Verification items for the finished model (mm, model axes). A direction names the side the tool comes from. Round coordinates to 2 decimals unless told otherwise and drop trailing zeros. Write each loop counter-clockwise with the first axis right and the second up, starting at its lowest first coordinate (ties: lowest second). Pieces come first, ordered by that corner, then holes. Notation, with made-up numbers: M 18,79 L 71,79 A12 ccw 71,83 Z; hole C 37,-33 d4. An arc over 180 degrees is marked long. One line per question, with ' | ' between items.
from build123d import *

# Parameters (mm, degrees)
SKETCH1_R           = 10
BOSS_EXTRUDE1_DEPTH = 4
SKETCH2_W           = 80
SKETCH2_H           = 30
BOSS_EXTRUDE2_DEPTH = 4
SKETCH5_W           = 15
SKETCH5_H           = 25.341978046
SKETCH5_R           = 3.5
BOSS_EXTRUDE3_DEPTH = 4
CUT_EXTRUDE1_DEPTH  = 5
SKETCH7_R           = 3.25
CUT_EXTRUDE2_DEPTH  = 5
LPATTERN1_COUNT     = 4
LPATTERN1_PITCH     = 12
SKETCH8_W           = 65
SKETCH8_H           = 10
BOSS_EXTRUDE4_DEPTH = 4
SKETCH9_R           = 1.175
CUT_EXTRUDE3_DEPTH  = 4
SKETCH10_W          = 10
SKETCH10_H          = 25
BOSS_EXTRUDE5_DEPTH = 4
SKETCH11_R          = 1.175
CUT_EXTRUDE4_DEPTH  = 4
SKETCH12_R          = 1
CUT_EXTRUDE5_DEPTH  = 5
CIRPATTERN1_COUNT   = 4
SKETCH13_R          = 3.5
CUT_EXTRUDE6_DEPTH  = 5
FILLET1_R           = 2


with BuildPart() as part:
    # Sketch1 → Boss-Extrude1 (new body)
    with BuildSketch(Plane(origin=(0, 0, 0), x_dir=(1, 0, 0), z_dir=(0, 1, 0))):
        Circle(SKETCH1_R)
    extrude(amount=BOSS_EXTRUDE1_DEPTH)

    # Sketch2 → Boss-Extrude2 (add)
    with BuildSketch(Plane(origin=(0, 0, 0), x_dir=(1, 0, 0), z_dir=(0, 1, 0))):
        with Locations((-40, 0)):
            Rectangle(SKETCH2_W, SKETCH2_H)
        Polygon((7.453553273, 6.666674104), (7.453553273, -6.666674104), (0, -15), (0, 15), align=None)
    extrude(amount=BOSS_EXTRUDE2_DEPTH)

    # Sketch5 → Boss-Extrude3 (add)
    with BuildSketch(Plane(origin=(0, 0, 0), x_dir=(1, 0, 0), z_dir=(0, 1, 0))):
        with Locations((-19.25, 27.670989023)):
            Rectangle(SKETCH5_W, SKETCH5_H)
        with Locations((-19.25, 33.341978046)):
            Circle(SKETCH5_R, mode=Mode.SUBTRACT)
    extrude(amount=BOSS_EXTRUDE3_DEPTH)

    # Sketch6 → Cut-Extrude1 (cut, through all)
    with BuildSketch(Plane(origin=(0, 4, 0), x_dir=(1, 0, 0), z_dir=(0, 1, 0))):
        with BuildLine():
            Line((-20.85, 24.912482213), (-20.514335664, 26.680907912))
            ThreePointArc((-20.514335664, 26.680907912), (-19.88495846, 26.591775993), (-19.25, 26.561978046))
            Line((-19.25, 26.561978046), (-19.25, 24.761978046))
            ThreePointArc((-19.25, 24.761978046), (-20.053531503, 24.799686952), (-20.85, 24.912482213))
        make_face()
    cut_extrude1 = extrude(amount=-CUT_EXTRUDE1_DEPTH, mode=Mode.SUBTRACT)

    # Mirror1: Cut-Extrude1 across plane
    add(cut_extrude1.mirror(Plane.ZY.offset(19.25)), mode=Mode.SUBTRACT)

    # Sketch7 → Cut-Extrude2 (cut, through all)
    with BuildSketch(Plane(origin=(0, 4, 0), x_dir=(1, 0, 0), z_dir=(0, 1, 0))):
        with Locations((-72, 0)):
            Circle(SKETCH7_R)
    cut_extrude2 = extrude(amount=-CUT_EXTRUDE2_DEPTH, mode=Mode.SUBTRACT)

    # LPattern1: Cut-Extrude2 ×4
    with Locations(*[(i * LPATTERN1_PITCH, 0, 0) for i in range(1, LPATTERN1_COUNT)]):
        add(cut_extrude2, mode=Mode.SUBTRACT)

    # Sketch8 → Boss-Extrude4 (add)
    with BuildSketch(Plane(origin=(0, 0, 0), x_dir=(1, 0, 0), z_dir=(0, 1, 0))):
        with Locations((20.75, 27)):
            Rectangle(SKETCH8_W, SKETCH8_H)
    extrude(amount=BOSS_EXTRUDE4_DEPTH)

    # Sketch9 → Cut-Extrude3 (cut)
    with BuildSketch(Plane(origin=(0, 4, 0), x_dir=(1, 0, 0), z_dir=(0, 1, 0))):
        with Locations((40.75, 26)):
            Circle(SKETCH9_R)
        with BuildLine():
            ThreePointArc((50.718101372, 30.374564563), (51.56619893, 27.22869882), (51.445333625, 23.97276081))
            ThreePointArc((51.445333625, 23.97276081), (50.22276081, 22.804666375), (49.054666375, 24.02723919))
            ThreePointArc((49.054666375, 24.02723919), (49.251093716, 26.76855347), (48.566204822, 29.430191102))
            ThreePointArc((48.566204822, 29.430191102), (49.169966366, 30.978326108), (50.718101372, 30.374564563))
        make_face()
    extrude(amount=-CUT_EXTRUDE3_DEPTH, mode=Mode.SUBTRACT)

    # Sketch10 → Boss-Extrude5 (add)
    with BuildSketch(Plane(origin=(0, 0, 0), x_dir=(1, 0, 0), z_dir=(0, 1, 0))):
        Polygon((-60, -55), (-60, -40), (-50, -40), align=None)
        with Locations((-55, -27.5)):
            Rectangle(SKETCH10_W, SKETCH10_H)
        Polygon((-60, -40), (-70, -55), (-60, -55), align=None)
    extrude(amount=BOSS_EXTRUDE5_DEPTH)

    # Sketch11 → Cut-Extrude4 (cut)
    with BuildSketch(Plane(origin=(0, 4, 0), x_dir=(1, 0, 0), z_dir=(0, 1, 0))):
        with Locations((-57.211102551, -43.605551275)):
            Circle(SKETCH11_R)
        with BuildLine():
            ThreePointArc((-61.363573117, -53.4398084), (-63.3936658, -52.307938113), (-65.130655612, -50.763505195))
            ThreePointArc((-65.130655612, -50.763505195), (-65.046826198, -49.103920117), (-63.387241121, -49.187749531))
            ThreePointArc((-63.387241121, -49.187749531), (-62.032633141, -50.392190191), (-60.449446107, -51.27488997))
            ThreePointArc((-60.449446107, -51.27488997), (-59.824050397, -52.81441269), (-61.363573117, -53.4398084))
        make_face()
    extrude(amount=-CUT_EXTRUDE4_DEPTH, mode=Mode.SUBTRACT)

    # Sketch12 → Cut-Extrude5 (cut, through all)
    with BuildSketch(Plane(origin=(0, 4, 0), x_dir=(1, 0, 0), z_dir=(0, 1, 0))):
        with Locations((7.1, 3.4)):
            Circle(SKETCH12_R)
        with Locations((7.1, -3.4)):
            Circle(SKETCH12_R)
        with Locations((7.1, 0)):
            Circle(SKETCH12_R)
    cut_extrude5 = extrude(amount=-CUT_EXTRUDE5_DEPTH, mode=Mode.SUBTRACT)

    # CirPattern1: Cut-Extrude5 ×4 about axis
    cirpattern1_axis = Axis((0, 0, 0), (0, 1, 0))
    for i in range(1, CIRPATTERN1_COUNT):
        add(cut_extrude5.rotate(cirpattern1_axis, i * 360 / CIRPATTERN1_COUNT), mode=Mode.SUBTRACT)

    # Sketch13 → Cut-Extrude6 (cut, through all)
    with BuildSketch(Plane(origin=(0, 4, 0), x_dir=(1, 0, 0), z_dir=(0, 1, 0))):
        Circle(SKETCH13_R)
    extrude(amount=-CUT_EXTRUDE6_DEPTH, mode=Mode.SUBTRACT)

    # Fillet1
    fillet1_edges = [part.edges().sort_by_distance(p)[0] for p in [
        (-11.75, 2, -32),
        (-11.75, 2, -22),
        (-60, 2, 15),
        (-60, 2, 40),
        (-70, 2, 55),
        (-60, 2, 55),
        (-50, 2, 40),
        (-50, 2, 15),
        (-11.75, 2, -15),
    ]]
    fillet(fillet1_edges, radius=FILLET1_R)


solid = part.part
1. Thickness scan on line 1 (Z direction, x = 7.1, y = 2.2); line 2 (X direction, y = 2.65, z = -7.1); line 3 (X direction, y = 2.8, z = -26) (3 decimals). Record the ranges inside material, lowest first.
Results:
line 1: z = -32 to -22, -7.06 to -4.4, -2.4 to -1, 1 to 2.4, 4.4 to 7.06 | line 2: x = -80 to -4.4, -2.4 to -1, 1 to 2.4, 4.4 to 7.07 | line 3: x = -26.75 to -20.644, -17.856 to 39.575, 41.925 to 49.286, 51.636 to 53.25
2. Tool access check on faces 4 (the face through (51.56, 2.03, -27.27)), 5 (the face through (21, 2, -22)), 6 (the face through (-24, 2, 15)), 7 (the face through (-64, 2, 46)), 8 (the face through (-26.75, 2, -27)). Record the directions out of +Z, -Z, +X, -X, +Y, -Y that give a thin tool (end or side, any length) a straight path to the whole face; none if there is none.
Results:
face 4: +Y, -Y | face 5: +X, +Y, -Y | face 6: +Z, +X, +Y, -Y | face 7: -X, +Y, -Y | face 8: -Z, -X, +Y, -Y
3. Go/stop test with flat-tipped pins: P1, Ø1, axis at y = 2, z = -11, coming from the +X side; P2, Ø6, axis at x = -33, z = -9, coming from the -Y side; P3, Ø1.2, axis at x = 14.5, y = 2.5, coming from the -Z side; P4, Ø2, axis at y = 2.5, z = 28, coming from the -X side. Record where each tip stops, or that it passes through.
Results:
P1: stops at x = 4.02 | P2: stops at y = 0 | P3: stops at z = -32 | P4: stops at x = -60
4. Mould release check, pull along X, two halves, no side actions. Record for faces 1 (the face through (-68.04, 2.03, 53.92)), 2 (the face through (-64, 2, 55)), 3 (the face through (3.233, 2.028, 1.341)): pulls with the +X half, pulls with the -X half, needs draft (parallel to the pull), parting line crosses it, or undercut.
Results:
face 1: pulls with the -X half | face 2: needs draft | face 3: undercut
5. Section check B-B, the plane y = 2.7. Count the separate pieces of the cut face and the enclosed holes in it, then the cut area to 3 significant figures.
Results:
separate pieces: 1 | enclosed holes: 23 | area: 3,720 mm2
6. Section check A-A, the plane z = 19. Record the cut outline in (x, y), then the cut area to 3 significant figures.
Results:
outline: M -60,0 L -50,0 L -50,4 L -60,4 Z | area: 40.0 mm2
